Autodesk Inventor part; units mm, degrees
ref_plane "YZ Plane" through (0, 0, 0) normal (1, 0, 0) x (0, 1, 0)
ref_plane "XZ Plane" through (0, 0, 0) normal (0, 1, 0) x (-1, 0, 0)
ref_plane "XY Plane" through (0, 0, 0) normal (0, 0, 1) x (1, 0, 0)
sketch "スケッチ1" plane through (0, 0, 0) normal (0, 0, 1) x (1, 0, 0)
  line L0 (-30, 30) -> (30, 30)
  line L1 (30, 30) -> (30, -30)
  line L2 (30, -30) -> (-30, -30)
  line L3 (-30, -30) -> (-30, 30)
  line L4 (-30, 30) -> (30, -30) construction
  line L5 (30, 30) -> (-30, -30) construction
  line L6 (-28, 28) -> (28, 28)
  line L7 (28, 28) -> (28, -28)
  line L8 (28, -28) -> (-28, -28)
  line L9 (-28, -28) -> (-28, 28)
  line L10 (-28, 28) -> (28, -28) construction
  line L11 (28, 28) -> (-28, -28) construction
  point P0 (0, 0)
  dimension "d0" = 60
  dimension "d1" = 60
  dimension "d2" = 56
  dimension "d3" = 56
extrude "押し出し1" add sketch "スケッチ1" along normal blind 80
sketch "スケッチ2" plane through (0, 0, 80) normal (0, 0, 1) x (1, 0, 0)
  line L0 (30, 30) -> (30, -30)
  line L1 (-30, -30) -> (30, -30)
  line L2 (30, -30) -> (30, -28)
  line L3 (30, -28) -> (-30, -28)
  line L4 (-30, -28) -> (-30, -30)
  point P0 (0, 0)
  dimension "d6" = 2
extrude "押し出し2" cut sketch "スケッチ2" against normal blind 100
sketch "スケッチ3" plane through (30, 30, 80) normal (1, 0, 0) x (0, 0, -1)
  line L0 (0, -58) -> (0, 0)
  line L1 (80, 0) -> (80, -58)
  line L2 (80, 0) -> (0, 0)
  point P0 (80, -30)
  point P1 (10, -7)
  point P2 (70, -7)
  dimension "d9" = 60
  dimension "d10" = 10
  dimension "d11" = 10
  dimension "d12" = 7
  dimension "d13" = 7
hole "穴1" at (30, 23, 70) at (30, 23, 10) direction (-1, 0, 0) diameter 3.2 end through all
sketch "スケッチ4" plane through (-30, 30, 0) normal (-1, 0, 0) x (0, 0, 1)
  line L0 (0, 0) -> (80, 0)
  line L1 (80, 0) -> (80, -58)
  point P0 (0, -30)
  point P1 (61.25, -52)
  point P2 (18.75, -52)
  dimension "d21" = 52
  dimension "d22" = 42.5
  dimension "d23" = 18.75
hole "穴2" at (-30, -22, 61.25) at (-30, -22, 18.75) direction (1, 0, 0) diameter 3.2 depth 8 tip angle 118
properties part number "Square pillar" material "アルミニウム 6061"
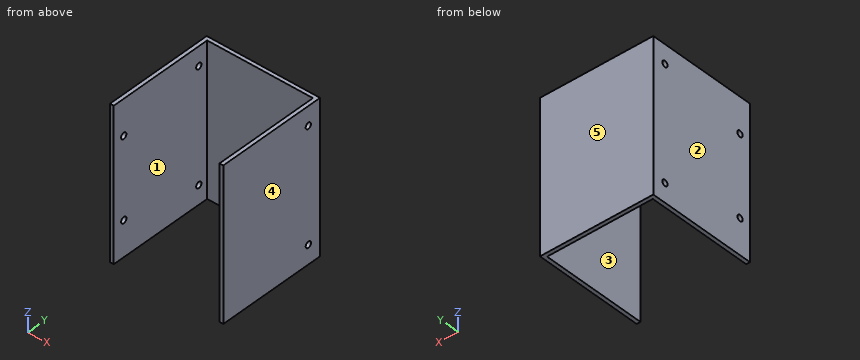
Source: CAD feature listing. Evaluate the final solid. Frame: model axes, mm. Face numbers are marked on the shaded views. A direction names the side the tool comes from. Round coordinates to 2 decimals unless told otherwise and drop trailing zeros. Write each loop counter-clockwise with the first axis right and the second up, starting at its lowest first coordinate (ties: lowest second). Pieces come first, ordered by that corner, then holes. Notation, with made-up numbers: (61.5, 41.5) - (79.5, 41.5) arc R15 ccw to (79.5, 64.5) - close; hole circle Ø1 at (37.25, 67.5). An arc over 180 degrees is marked (long way). Use CSV: the item, a comma, the result in double quotes. Start each with the question number.
(1) Cut plane C-C, the plane z = 70. Return loops of the section in (x, y), and give its area (3 significant figures).
(2) Cut plane D-D, the plane z = 27. Return loops of the section in (x, y).
(3) Cut plane B-B, the plane y = 14.5. Return loops of the section in (x, z).
(4) Mould query, pull axis X, two halves, no side actions, for the marked faces 3, 4 and 5. Classes: pulls with the +X half, pulls with the -X half, needs draft (parallel to the pull), parting line crosses it, or undercut.
(5) First-contact query: pin 1 Ø12 at (x, y) = (0, 17) entering from +Z; pin 2 Ø3 at (x, z) = (23, 33) entering from -Y. Flat tips, straight axial feed; report the tip coordinate or a pass-through.
(6) Cut plane A-A, the plane z = 61.25. Return loops of the section in (x, y), and give its area (3 significant figures).
(7) Set-up query: the marked faces 1 and 2. Return all of +Z, -Z, +X, -X, +Y, -Y with unobstructed straight access to the full face (end or side cutting, diameter ignored); none if empty.
(8) Material intervals for probe 1 along Z at (x, y) = (-29.55, 23); probe 2 along X at (y, z) = (-19.5, 21.5); probe 3 along Y at (x, z) = (29.5, 70), sorted ascending. Write a range as [from, to].
Geometry says:
1,outline,"(-30, -28) - (-28, -28) - (-28, 21.4) - (-30, 21.4) - close; (-30, 24.6) - (-28, 24.6) - (-28, 28) - (28, 28) - (28, 24.6) - (30, 24.6) - (30, 30) - (-30, 30) - close; (28, -28) - (30, -28) - (30, 21.4) - (28, 21.4) - close"
1,area,"331 mm²"
2,outline,"(-30, -28) - (-28, -28) - (-28, 28) - (28, 28) - (28, -28) - (30, -28) - (30, 30) - (-30, 30) - close"
3,outline,"(-30, 0) - (-28, 0) - (-28, 80) - (-30, 80) - close; (28, 0) - (30, 0) - (30, 80) - (28, 80) - close"
4,face 3,"undercut"
4,face 4,"pulls with the +X half"
4,face 5,"needs draft"
5,pin 1,"through"
5,pin 2,"y = 28"
6,outline,"(-30, -28) - (-28, -28) - (-28, -23.6) - (-30, -23.6) - close; (-30, -20.4) - (-28, -20.4) - (-28, 28) - (28, 28) - (28, -28) - (30, -28) - (30, 30) - (-30, 30) - close"
6,area,"338 mm²"
7,face 1,"+Z, -Z, -Y"
7,face 2,"+Z, -Z, -X, +Y, -Y"
8,probe 1,"[0, 8.4], [11.6, 68.4], [71.6, 80]"
8,probe 2,"[-30, -28], [28, 30]"
8,probe 3,"[-28, 21.4], [24.6, 30]"
